```python
from build123d import *

# Parameters (mm, degrees)
F0_R     = 2.54
F0_R_2   = 1.27
F1_DEPTH = 2.54
F2_DEPTH = 25.4
F3_DEPTH = 50.8


with BuildPart() as f1:
    # F0 (on Top) → F1 (new body)
    with BuildSketch(Plane.XY):
        Polygon((-47.093086, -27.160453), (-47.093086, -34.780453), (-39.473086, -34.780453), (-31.853086, -34.780453), (-31.853086, -27.160453), (-39.473086, -27.160453), align=None)
        with Locations((-43.283086, -31.007911)):
            Circle(F0_R, mode=Mode.SUBTRACT)
        with Locations((-35.700362, -31.007911)):
            Circle(F0_R, mode=Mode.SUBTRACT)
        with Locations((-43.283086, -31.007911)):
            Circle(F0_R)
        with Locations((-43.283086, -31.007911)):
            Circle(F0_R_2, mode=Mode.SUBTRACT)
        with Locations((-43.283086, -31.007911)):
            Circle(F0_R_2)
        with Locations((-35.700362, -31.007911)):
            Circle(F0_R)
        with Locations((-35.700362, -31.007911)):
            Circle(F0_R_2, mode=Mode.SUBTRACT)
        with Locations((-35.700362, -31.007911)):
            Circle(F0_R_2)
    extrude(amount=-F1_DEPTH)

    # F0 (on Top) → F2 (join)
    with BuildSketch(Plane.XY):
        with Locations((-43.283086, -31.007911)):
            Circle(F0_R)
        with Locations((-43.283086, -31.007911)):
            Circle(F0_R_2, mode=Mode.SUBTRACT)
        with Locations((-35.700362, -31.007911)):
            Circle(F0_R)
        with Locations((-35.700362, -31.007911)):
            Circle(F0_R_2, mode=Mode.SUBTRACT)
    extrude(amount=F2_DEPTH)

    # F0 (on Top) → F3 (join)
    with BuildSketch(Plane.XY):
        with Locations((-43.283086, -31.007911)):
            Circle(F0_R_2)
        with Locations((-35.700362, -31.007911)):
            Circle(F0_R_2)
    extrude(amount=F3_DEPTH)


solid = f1.part
```
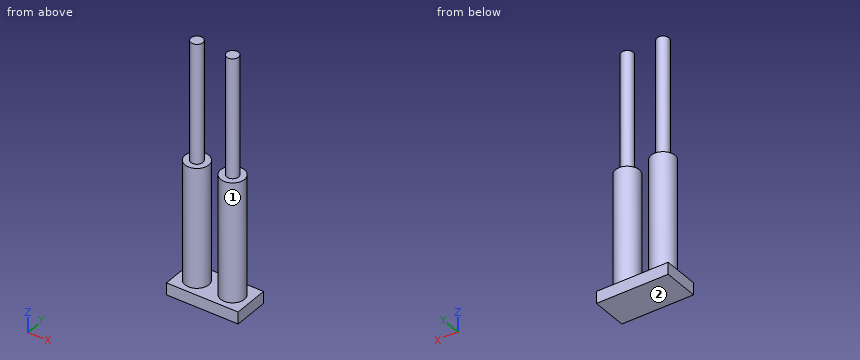
Work out the finished part from the listing and answer in its coordinate system (mm). Face numbers are marked on the shaded views. Give positions to 0.01 mm unless a question says otherwise; leave off trailing zeros. Loops run counter-clockwise (first coordinate to the right, second up) from the corner with the lowest first, then second, coordinate; pieces in that order, holes last. Notation, with made-up numbers: (36, -20.75) - (43, -20.75) arc R36 ccw to (43, 13.25) - close; hole circle Ø10 at (-16.5, 45.25). An arc over 180 degrees is marked (long way). One line per question, with ' | ' between items.
(1) The part is cut by section B-B (x = -42.75). Write down the section's boundary in (y, z), then the cut area to 3 significant figures.
Recorded:
outline: (-34.78, -2.54) - (-27.16, -2.54) - (-27.16, 0) - (-28.52, 0) - (-28.52, 25.4) - (-29.86, 25.4) - (-29.86, 50.8) - (-32.16, 50.8) - (-32.16, 25.4) - (-33.49, 25.4) - (-33.49, 0) - (-34.78, 0) - close | area: 204 mm²
(2) The part is cut by section A-A (y = -30.25). Write down the section's boundary in (x, z), then the cut area to 3 significant figures.
Recorded:
outline: (-47.09, -2.54) - (-31.85, -2.54) - (-31.85, 0) - (-33.28, 0) - (-33.28, 25.4) - (-34.68, 25.4) - (-34.68, 50.8) - (-36.72, 50.8) - (-36.72, 25.4) - (-38.12, 25.4) - (-38.12, 0) - (-40.86, 0) - (-40.86, 25.4) - (-42.26, 25.4) - (-42.26, 50.8) - (-44.3, 50.8) - (-44.3, 25.4) - (-45.71, 25.4) - (-45.71, 0) - (-47.09, 0) - close | area: 389 mm²
(3) The mould has two halves that part along X. Classify the marked faces 1 and 2: +X half, -X half, draft (parallel to the pull), parting line (faces both ways), or undercut.
Recorded:
face 1: undercut | face 2: draft
(4) Straight lines are drawn through the part: probe 1 along Z at (x, y) = (-40, -34.25); probe 2 along Z at (x, y) = (-42, -31.75); probe 3 along X at (y, z) = (-32.5, 13). For each, find the intervals that lie inside material, in ascending order.
Recorded:
probe 1: z = -2.54 to 0 | probe 2: z = -2.54 to 25.4 | probe 3: x = -45.34 to -41.23, -37.76 to -33.64
(5) The part is cut by section C-C (z = 10). Write down the section's boundary in (x, y), then the cut area to 3 significant figures.
Recorded:
outline: circle Ø5.08 at (-43.28, -31.01); circle Ø5.08 at (-35.7, -31.01) | area: 40.5 mm²
(6) Each of these flat-tipped pins is pushed along its axis until it touches: pin 1 Ø1 at (x, z) = (-39.5, 10.5) entering from -Y; pin 2 Ø3 at (x, y) = (-38.5, -30.5) entering from +Z; pin 3 Ø5 at (x, z) = (-33.5, 34.5) entering from +Y; pin 4 Ø1.5 at (x, z) = (-36, 20) entering from +Y. Where does it stop, or does it pass through?
Recorded:
pin 1: passes through | pin 2: stops at z = 25.4 | pin 3: stops at y = -29.74 | pin 4: stops at y = -28.47
(7) The part is cut by section D-D (z = 29.5). Write down the section's boundary in (x, y).
Recorded:
outline: circle Ø2.54 at (-43.28, -31.01); circle Ø2.54 at (-35.7, -31.01)
